Verification items for the finished model (mm, model axes). Face numbers are marked on the shaded views. A direction names the side the tool comes from. Coordinates: 2 decimals unless noted, no trailing zeros. Loops run counter-clockwise (first coordinate to the right, second up) from the corner with the lowest first, then second, coordinate; pieces in that order, holes last. Notation, with made-up numbers: (55.5, -36) - (83.5, -36) arc R7 cw to (83.5, -32) - close; hole circle Ø7 at (-15.75, 23). An arc over 180 degrees is marked (long way). Answer as CSV lines item,"result". Start each with the question number.
1. Set-up check for the marked faces 1, 2, 3 and 4: record each of +Z, -Z, +X, -X, +Y, -Y from which the full face is reachable in a straight line by a thin tool's end or side.
2. Gauge pin test, flat ends, axial feed: P1, Ø10, axis at x = -0.5, z = 0.5, coming from the +Y side (3 decimals); P2, Ø3, axis at x = -19.5, z = 12, coming from the +Y side; P3, Ø4, axis at x = 20.5, y = 24, coming from the -Z side; P4, Ø12, axis at x = -20, y = 14.5, coming from the +Z side. Record the tip position at first contact, or that the pin passes through.
3. Cross-section at B-B (x = 17). Enter the section's corners in (y, z).
4. Material ranges on line 1 (X direction, y = -2.75, z = 0) (3 decimals); line 2 (X direction, y = 20.5, z = 8); line 3 (Z direction, x = 0, y = 0.75) (3 decimals), recorded low to high. Write a range as [from, to].
5. Cross-section at A-A (y = 14). Enter the section's corners in (x, z) (3 decimals).
6. Cross-section at C-C (y = -10). Enter the section's corners in (x, z) (3 decimals), plus the area to 3 significant figures.
7. Release check for a two-part mould opening along Z. For the marked faces 5, 6, 7 and 8 record: pulls with the +Z half, pulls with the -Z half, needs draft (parallel to the pull), parting line crosses it, or undercut.
```python
from build123d import *

# Parameters (mm, degrees)
SKETCH1_W           = 51.355839692
SKETCH1_H           = 51.355839692
BOSS_EXTRUDE1_DEPTH = 21.828125
FILLET1_R           = 6.35
SHELL1_T            = -3.175
SKETCH2_R           = 15.875
BOSS_EXTRUDE2_DEPTH = 12.7
SKETCH3_W           = 6.35
SKETCH3_H           = 45.005839692
BOSS_EXTRUDE3_DEPTH = 18.653125
SKETCH4_R           = 4.7625
BOSS_EXTRUDE4_DEPTH = 12.7
CUT_EXTRUDE1_DEPTH  = 25.4
SKETCH6_R           = 1.966828055
BOSS_EXTRUDE5_DEPTH = 0.79375
FILLET2_R           = 3.175
FILLET3_R           = 3.175
SKETCH8_R           = 13.335
CUT_EXTRUDE2_DEPTH  = 12.7
CUT_EXTRUDE3_START  = -6.35
SKETCH9_R           = 0.1
CUT_EXTRUDE3_DEPTH  = 8.89
CIRPATTERN1_COUNT   = 4
CHAMFER4_SIZE       = 0.762
CHAMFER5_SIZE       = 0.508


with BuildPart() as part:
    # Sketch1 → Boss-Extrude1 (new body)
    with BuildSketch(Plane(origin=(0, 0, 0), x_dir=(1, 0, 0), z_dir=(0, 1, 0))):
        Rectangle(SKETCH1_W, SKETCH1_H)
    extrude(amount=BOSS_EXTRUDE1_DEPTH)

    # Fillet1
    fillet1_edges = [part.edges().sort_by_distance(p)[0] for p in [
        (25.677919846, 10.9140625, -25.677919846),
        (25.677919846, 10.9140625, 25.677919846),
        (-25.677919846, 10.9140625, 25.677919846),
        (-25.677919846, 10.9140625, -25.677919846),
    ]]
    fillet(fillet1_edges, radius=FILLET1_R)

    # Shell1
    shell1_openings = [part.faces().sort_by_distance(p)[0] for p in [
        (0, 21.828125, 0),
    ]]
    offset(amount=SHELL1_T, openings=shell1_openings, kind=Kind.INTERSECTION)

    # Sketch2 → Boss-Extrude2 (add)
    with BuildSketch(Plane.XZ):
        with Locations(Location((0, 0, 0), (0, 0, 270))):
            Circle(SKETCH2_R)
    extrude(amount=BOSS_EXTRUDE2_DEPTH)

    # Sketch3 → Boss-Extrude3 (add)
    with BuildSketch(Plane(origin=(0, 3.175, 0), x_dir=(1, 0, 0), z_dir=(0, 1, 0))):
        with Locations((19.327919846, 0)):
            Rectangle(SKETCH3_W, SKETCH3_H)
    extrude(amount=BOSS_EXTRUDE3_DEPTH)

    # Sketch4 → Boss-Extrude4 (add, symmetric)
    with BuildSketch(Plane.XY):
        with Locations((20.915419846, 21.828125)):
            Circle(SKETCH4_R)
    extrude(amount=BOSS_EXTRUDE4_DEPTH, both=True)

    # Sketch5 → Cut-Extrude1 (cut)
    with BuildSketch(Plane.XY.offset(12.7)):
        with BuildLine():
            ThreePointArc((22.502919846, 24.209375), (22.037951861, 25.331907015), (20.915419846, 25.796875))
            Line((20.915419846, 25.796875), (20.915419846, 22.621875))
            ThreePointArc((20.915419846, 22.621875), (22.037951861, 23.086842985), (22.502919846, 24.209375))
        make_face()
        with BuildLine():
            Line((20.915419846, 22.621875), (20.915419846, 25.796875))
            ThreePointArc((20.915419846, 25.796875), (19.327919846, 24.209375), (20.915419846, 22.621875))
        make_face()
    extrude(amount=-CUT_EXTRUDE1_DEPTH, mode=Mode.SUBTRACT)

    # Sketch6 → Boss-Extrude5 (add)
    with BuildSketch(Plane.XY.offset(12.7)):
        with Locations((20.915419846, 24.209375)):
            Circle(SKETCH6_R)
    extrude(amount=-BOSS_EXTRUDE5_DEPTH)

    # Fillet2
    fillet2_edges = [part.edges().sort_by_distance(p)[0] for p in [
        (16.152919846, 12.5015625, 22.502919846),
        (16.152919846, 12.5015625, -22.502919846),
    ]]
    fillet(fillet2_edges, radius=FILLET2_R)

    # Fillet3
    fillet3_edges = [part.edges().sort_by_distance(p)[0] for p in [
        (16.152919846, 3.175, 0),
        (-3.175, 3.175, -22.502919846),
        (15.222983876, 3.175, -21.572983876),
        (15.222983876, 3.175, 21.572983876),
        (-22.502919846, 3.175, 0),
        (-3.175, 3.175, 22.502919846),
        (-21.572983876, 3.175, 21.572983876),
        (-21.572983876, 3.175, -21.572983876),
    ]]
    fillet(fillet3_edges, radius=FILLET3_R)

    # Sketch8 → Cut-Extrude2 (cut)
    with BuildSketch(Plane.XZ.offset(12.7)):
        with Locations(Location((0, 0, 0), (0, 0, 270))):
            Circle(SKETCH8_R)
    extrude(amount=-CUT_EXTRUDE2_DEPTH, mode=Mode.SUBTRACT)

    # Sketch9 → Cut-Extrude3 (cut)
    with BuildSketch(Plane(origin=(0, 0, 0), x_dir=(1, 0, 0), z_dir=(0, 1, 0)).offset(CUT_EXTRUDE3_START)):
        with Locations(Location((-14.605, 0, 0), (0, 0, 270))):
            Circle(SKETCH9_R)
    cut_extrude3 = extrude(amount=CUT_EXTRUDE3_DEPTH, mode=Mode.SUBTRACT)

    # CirPattern1: Cut-Extrude3 ×4 about axis
    cirpattern1_axis = Axis((0, 0, 0), (0, 1, 0))
    for i in range(1, CIRPATTERN1_COUNT):
        add(cut_extrude3.rotate(cirpattern1_axis, i * 360 / CIRPATTERN1_COUNT), mode=Mode.SUBTRACT)

    # Chamfer4
    chamfer4_edges = [part.edges().sort_by_distance(p)[0] for p in [
        (0, 0, -25.677919846),
        (25.677919846, 0, 0),
        (0, 0, 25.677919846),
        (-25.677919846, 0, 0),
        (-23.818047907, 0, -23.818047907),
        (-23.818047907, 0, 23.818047907),
        (23.818047907, 0, 23.818047907),
        (23.818047907, 0, -23.818047907),
    ]]
    chamfer(chamfer4_edges, length=CHAMFER4_SIZE)

    # Chamfer5
    chamfer5_edges = [part.edges().sort_by_distance(p)[0] for p in [
        (0, -12.7, 13.335),
        (0, -12.7, 15.875),
    ]]
    chamfer(chamfer5_edges, length=CHAMFER5_SIZE)


solid = part.part
```
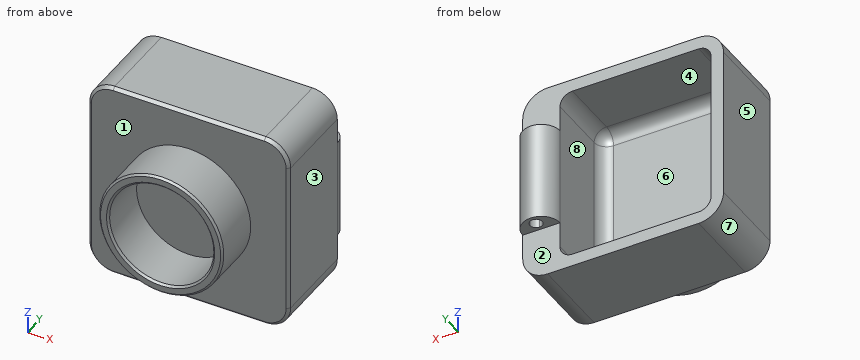
Values follow:
1,face 1,"-Y"
1,face 2,"-X, +Y"
1,face 3,"+Z, -Z, +X, +Y, -Y"
1,face 4,"+Y"
2,P1,"stops at y = 3.175"
2,P2,"stops at y = 3.65"
2,P3,"stops at z = -12.7"
2,P4,"stops at z = 25.68"
3,outline,"(0, -24.92) - (0.76, -25.68) - (21.83, -25.68) - (21.83, -12.7) - (24.54, -12.7) - (24.54, 12.7) - (21.83, 12.7) - (21.83, 25.68) - (0.76, 25.68) - (0, 24.92) - close"
4,line 1,"x = [-15.875, -14.705], [-14.505, -13.335], [13.335, 14.505], [14.705, 15.875]"
4,line 2,"x = [-25.68, -22.5], [16.15, 25.68]"
4,line 3,"z = [-25.666, -14.705], [-14.505, 14.505], [14.705, 25.666]"
5,outline,"(-25.678, -19.328) arc R6.35 ccw to (-19.328, -25.678) - (19.328, -25.678) arc R6.35 ccw to (25.678, -19.328) - (25.678, 19.328) arc R6.35 ccw to (19.328, 25.678) - (-19.328, 25.678) arc R6.35 ccw to (-25.678, 19.328) - close; hole (-22.503, -19.328) arc R3.175 ccw to (-19.328, -22.503) - (12.978, -22.503) arc R3.175 ccw to (16.153, -19.328) - (16.153, 19.328) arc R3.175 ccw to (12.978, 22.503) - (-19.328, 22.503) arc R3.175 ccw to (-22.503, 19.328) - close"
6,outline,"circle Ø31.75 at (0, 0); hole circle Ø26.67 at (0, 0)"
6,area,"233 mm²"
7,face 5,"needs draft"
7,face 6,"undercut"
7,face 7,"pulls with the -Z half"
7,face 8,"undercut"
